Geometry: see drawing. Coordinates: mm, zero at the bounding-box minimum. A direction names the side the tool comes from. Give positions to 0.01 mm unless a question says otherwise; leave off trailing zeros. Loops run counter-clockwise (first coordinate to the right, second up) from the corner with the lowest first, then second, coordinate; pieces in that order, holes last. Notation, with made-up numbers: (20.5, -8) -> (25.5, -8) arc R11 ccw to (25.5, 11) -> close; hole circle Ø1 at (-10.75, 88). An arc over 180 degrees is marked (long way). Return JSON: item names as keys, results as strings. Group by question number.
(1) Cut plane B-B on z = 28.75. Give the number of separate pieces and of enclosed holes in the cut face, then the cut area to 3 significant figures.
(2) Access query for the marked faces 1 and 2. Directions: +Z, -Z, +X, -X, +Y, -Y. A direction counts if a zero-diameter tool reaches every point of the face in a straight line with its end or side. Return the directions, or none.
(3) Cut plane C-C on y = 9.5. Return loops of the section in (x, z).
(4) Pin query (flat end, axial travel): pin 1 (4 mm diameter, centred on x = 8.5, z = 30, fed in from +Y). Return the tip coordinate at first contact, or that it passes through.
(5) Draft query along X for the marked faces 3, 4, 5 and 6. Return one class per face: released by +X, released by -X, zero draft, split by the parting line, or undercut.
(6) Ray query, line 1 (X direction, y = 1.3, z = 28.75); line 2 (X direction, y = 0.4, z = 28.75); line 3 (X direction, y = 5.25, z = 23.5). Return the intervals inside material, ascending. Write a range as from..to.
(7) Cut plane D-D on x = 26.5. Return loops of the section in (y, z), then the cut area to 3 significant figures.
(8) Cut plane A-A on x = 38.35. Return loops of the section in (y, z), then the cut area to 3 significant figures.
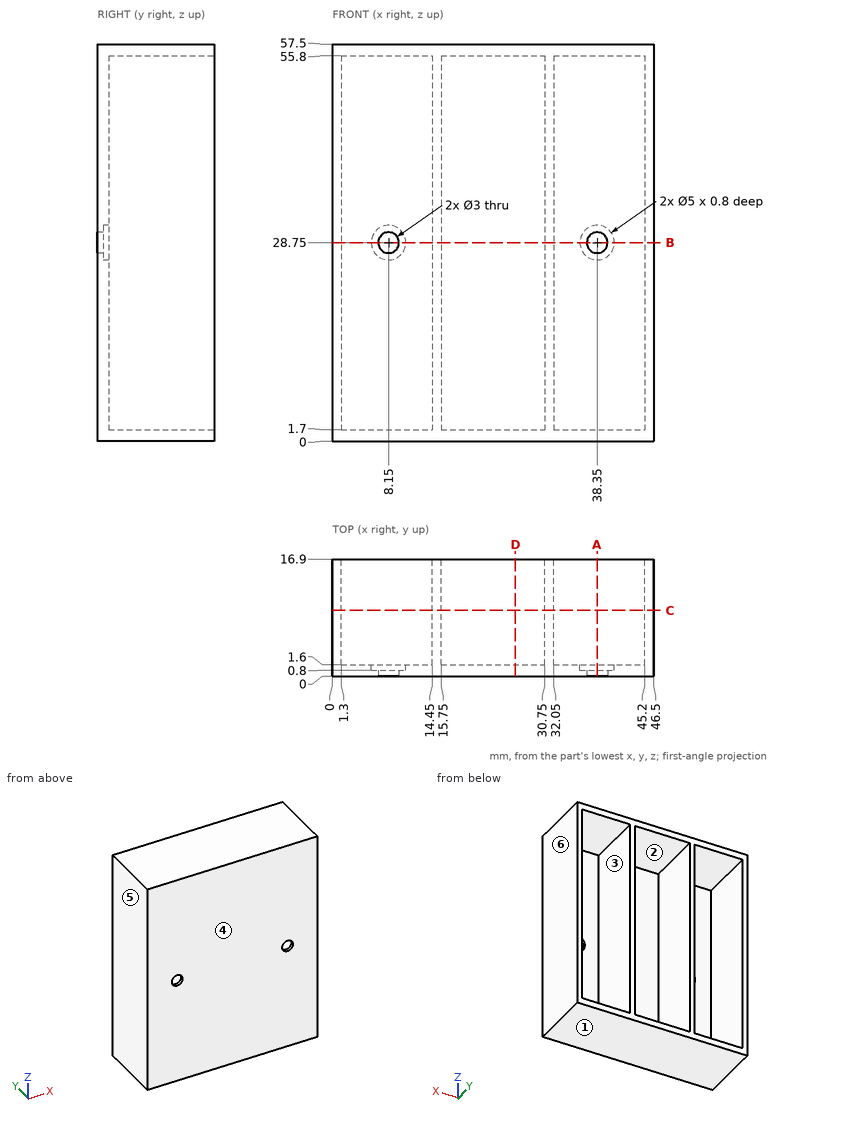
Answers:
{
 "1": {"separate pieces": "3", "enclosed holes": "0", "area": "141 mm²"},
 "2": {"face 1": "-Z, +X, -X, +Y, -Y", "face 2": "+Y"},
 "3": {"outline": "(0, 0) -> (46.5, 0) -> (46.5, 57.5) -> (0, 57.5) -> close; hole (1.3, 1.7) -> (14.45, 1.7) -> (14.45, 55.8) -> (1.3, 55.8) -> close; hole (15.75, 1.7) -> (30.75, 1.7) -> (30.75, 55.8) -> (15.75, 55.8) -> close; hole (32.05, 1.7) -> (45.2, 1.7) -> (45.2, 55.8) -> (32.05, 55.8) -> close"},
 "4": {"pin 1": "y = 1.6"},
 "5": {"face 3": "undercut", "face 4": "zero draft", "face 5": "released by -X", "face 6": "released by +X"},
 "6": {"line 1": "0..5.65, 10.65..35.85, 40.85..46.5", "line 2": "0..6.65, 9.65..36.85, 39.85..46.5", "line 3": "0..1.3, 14.45..15.75, 30.75..32.05, 45.2..46.5"},
 "7": {"outline": "(0, 0) -> (16.9, 0) -> (16.9, 1.7) -> (1.6, 1.7) -> (1.6, 55.8) -> (16.9, 55.8) -> (16.9, 57.5) -> (0, 57.5) -> close", "area": "144 mm²"},
 "8": {"outline": "(0, 0) -> (16.9, 0) -> (16.9, 1.7) -> (1.6, 1.7) -> (1.6, 26.25) -> (0.8, 26.25) -> (0.8, 27.25) -> (0, 27.25) -> close; (0, 30.25) -> (0.8, 30.25) -> (0.8, 31.25) -> (1.6, 31.25) -> (1.6, 55.8) -> (16.9, 55.8) -> (16.9, 57.5) -> (0, 57.5) -> close", "area": "138 mm²"}
}
